```python
from build123d import *

# Parameters (mm, degrees)
SKETCH2_R           = 23
BOSS_EXTRUDE1_DEPTH = 127
SKETCH3_R           = 13
BOSS_EXTRUDE2_DEPTH = 2
SKETCH4_R           = 4
BOSS_EXTRUDE3_DEPTH = 20
SKETCH8_R           = 2
CUT_EXTRUDE1_DEPTH  = 10
CUT_EXTRUDE2_DEPTH  = 12


with BuildPart() as part:
    # Sketch2 → Boss-Extrude1 (new body)
    with BuildSketch(Plane(origin=(0, 0, 0), x_dir=(1, 0, 0), z_dir=(0, 1, 0))):
        Circle(SKETCH2_R)
    extrude(amount=BOSS_EXTRUDE1_DEPTH)

    # Sketch3 → Boss-Extrude2 (add)
    with BuildSketch(Plane(origin=(0, 127, 0), x_dir=(1, 0, 0), z_dir=(0, 1, 0))):
        Circle(SKETCH3_R)
    extrude(amount=BOSS_EXTRUDE2_DEPTH)

    # Sketch4 → Boss-Extrude3 (add)
    with BuildSketch(Plane(origin=(0, 129, 0), x_dir=(1, 0, 0), z_dir=(0, 1, 0))):
        Circle(SKETCH4_R)
    extrude(amount=BOSS_EXTRUDE3_DEPTH)

    # Sketch8 → Cut-Extrude1 (cut)
    with BuildSketch(Plane(origin=(0, 127, 0), x_dir=(1, 0, 0), z_dir=(0, 1, 0))):
        with Locations((0, 18)):
            Circle(SKETCH8_R)
        with Locations((18, 0)):
            Circle(SKETCH8_R)
        with Locations((0, -18)):
            Circle(SKETCH8_R)
        with Locations((-18, 0)):
            Circle(SKETCH8_R)
    extrude(amount=-CUT_EXTRUDE1_DEPTH, mode=Mode.SUBTRACT)

    # Sketch10 → Cut-Extrude2 (cut)
    with BuildSketch(Plane(origin=(0, 149, 0), x_dir=(1, 0, 0), z_dir=(0, 1, 0))):
        Polygon((-84.712273825, 3.5), (-1.936491673, 3.5), (1.936491673, 3.5), (84.712273825, 3.5), (84.712273825, 169.051564304), (-84.712273825, 169.051564304), align=None)
    extrude(amount=-CUT_EXTRUDE2_DEPTH, mode=Mode.SUBTRACT)


solid = part.part
```
For this review, take the finished solid that the model builds, in its own axes (mm). A direction names the side the tool comes from. Give positions to 0.01 mm unless a question says otherwise; leave off trailing zeros. Order: outer loops, then holes, each group sorted by start corner. A loop starts at its lowest first (then second) coordinate and runs counter-clockwise, first axis right, second up.
1) The part is to be moulded in two halves that separate along X. For faces 1 (the face through (0, 149, 0)), 2 (the face through (0, 122, 16)), 3 (the face through (-0.867, 138.86, 3.905)), say which applies: released by +X, released by -X, zero draft, split by the parting line, or undercut.
2) Take a section at B-B (y = 121). Give the boundary of the cut face in (x, z).
3) For faces 4 (the face through (0, 0, 0)), 5 (the face through (18, 117, 0)), 6 (the face through (0, 143, -3.5)), list the 3-axis set-ups (+Z, -Z, +X, -X, +Y, -Y) from which the entire face can be reached by the end or side of a thin tool; tool diameter is ignored.
4) Take a section at D-D (y = 79.5). Give the boundary of the cut face in (x, z).
5) Take a section at A-A (x = 0). Give the boundary of the cut face in (y, z), then the cut area to 3 significant figures.
6) Take a section at C-C (z = 0). Give the boundary of the cut face in (x, y), then the cut area to 3 significant figures.
7) Insertion check: pin 1 (1.2 mm diameter, centred on x = 0.5, y = 146, fed in from -Z); pin 2 (4.5 mm diameter, centred on x = 17, z = -0.5, fed in from +Y); pin 3 (4 mm diameter, centred on y = 98, z = 11.5, fed in from -X). Each pin has a flat end and moves straight along its axis. Give the tip position at first contact, or say it passes through.
8) Wall thickness on line 1 (X direction, y = 119, z = 0); line 2 (Y direction, x = 0.5, z = -7.5): over which ranges is each line inside the solid? List them lowest first.
Derived:
1. face 1: zero draft
1. face 2: undercut
1. face 3: split by the parting line
2. outline: circle Ø46 at (0, 0); hole circle Ø4 at (-18, 0); hole circle Ø4 at (0, -18); hole circle Ø4 at (0, 18); hole circle Ø4 at (18, 0)
3. face 4: +Z, -Z, +X, -X, -Y
3. face 5: +Y
3. face 6: -Z, +X, -X, +Y
4. outline: circle Ø46 at (0, 0)
5. outline: (0, -23) - (127, -23) - (127, -20) - (117, -20) - (117, -16) - (127, -16) - (127, -13) - (129, -13) - (129, -4) - (137, -4) - (137, -3.5) - (149, -3.5) - (149, 4) - (129, 4) - (129, 13) - (127, 13) - (127, 16) - (117, 16) - (117, 20) - (127, 20) - (127, 23) - (0, 23) - close
5. area: 5,970 mm2
6. outline: (-23, 0) - (23, 0) - (23, 127) - (20, 127) - (20, 117) - (16, 117) - (16, 127) - (13, 127) - (13, 129) - (4, 129) - (4, 149) - (-4, 149) - (-4, 129) - (-13, 129) - (-13, 127) - (-16, 127) - (-16, 117) - (-20, 117) - (-20, 127) - (-23, 127) - close
6. area: 5,970 mm2
7. pin 1: stops at z = -3.5
7. pin 2: stops at y = 127
7. pin 3: stops at x = -20.95
8. line 1: x = -23 to -20, -16 to 16, 20 to 23
8. line 2: y = 0 to 129
